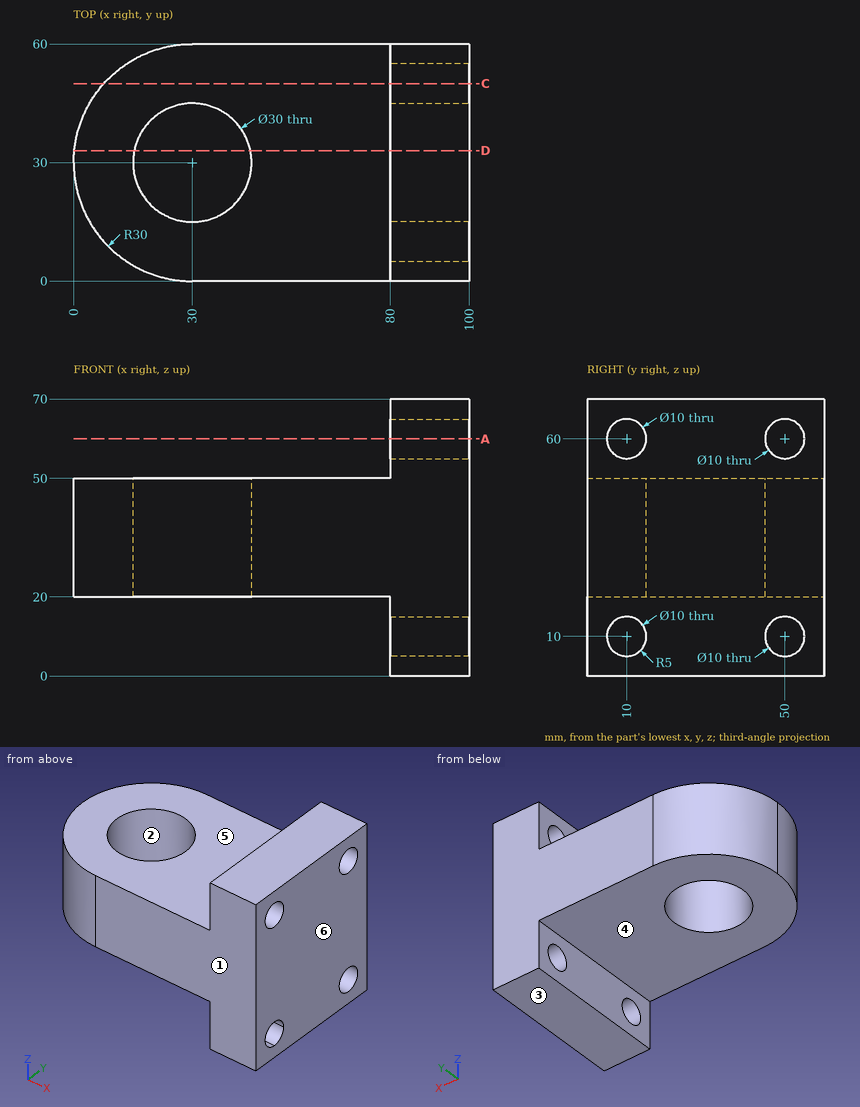
Check sheet for the drawn part. Datum: minimum x, y, z corner. Units: mm. A direction names the side the tool comes from. Coordinates: 2 decimals unless noted, no trailing zeros. Order: outer loops, then holes, each group sorted by start corner. A loop starts at its lowest first (then second) coordinate and runs counter-clockwise, first axis right, second up. Notation, with made-up numbers: (-11, 84.5) -> (8, 84.5) arc R29 cw to (8, 113.5) -> close; hole circle Ø11 at (21, 2). An arc over 180 degrees is marked (long way). Use a Markdown table: item, result. Add a question column.
1. Cross-section at D-D (y = 33). Enter the section's corners in (x, z), and give its area (3 significant figures).
2. Cross-section at A-A (z = 60). Enter the section's corners in (x, y).
3. Mould release check, pull along Y, two halves, no side actions. Record for the marked faces 1, 2 and 3: pulls with the +Y half, pulls with the -Y half, needs draft (parallel to the pull), parting line crosses it, or undercut.
4. Set-up check for the marked faces 4, 5 and 6: record each of +Z, -Z, +X, -X, +Y, -Y from which the full face is reachable in a straight line by a thin tool's end or side.
5. Go/stop test with flat-tipped pins: pin 1 Ø6 at (y, z) = (22, 7.5) entering from -X; pin 2 Ø6 at (x, y) = (54.5, 37) entering from +Z; pin 3 Ø16 at (y, z) = (10, 10) entering from +X; pin 4 Ø10 at (y, z) = (50, 52) entering from -X. Record where each tip stops, or that it passes through.
6. Cross-section at C-C (y = 50). Enter the section's corners in (x, z), and give its area (3 significant figures).
7. Material ranges on L1, parallel to Z at x = 92.5, y = 50; L2, parallel to Y at x = 30, z = 35; L3, parallel to X at y = 54.5, z = 7.5, recorded low to high.
Filled sheet:
| question | item | result |
|---|---|---|
| 1 | outline | (0.15, 20) -> (15.3, 20) -> (15.3, 50) -> (0.15, 50) -> close; (44.7, 20) -> (80, 20) -> (80, 0) -> (100, 0) -> (100, 70) -> (80, 70) -> (80, 50) -> (44.7, 50) -> close |
| 1 | area | 2,910 mm2 |
| 2 | outline | (80, 0) -> (100, 0) -> (100, 5) -> (80, 5) -> close; (80, 15) -> (100, 15) -> (100, 45) -> (80, 45) -> close; (80, 55) -> (100, 55) -> (100, 60) -> (80, 60) -> close |
| 3 | face 1 | pulls with the -Y half |
| 3 | face 2 | undercut |
| 3 | face 3 | needs draft |
| 4 | face 4 | -Z, -X, +Y, -Y |
| 4 | face 5 | +Z, -X, +Y, -Y |
| 4 | face 6 | +Z, -Z, +X, +Y, -Y |
| 5 | pin 1 | x = 80 |
| 5 | pin 2 | z = 50 |
| 5 | pin 3 | x = 100 |
| 5 | pin 4 | x = 4.26 |
| 6 | outline | (7.64, 20) -> (80, 20) -> (80, 15) -> (100, 15) -> (100, 55) -> (80, 55) -> (80, 50) -> (7.64, 50) -> close; (80, 0) -> (100, 0) -> (100, 5) -> (80, 5) -> close; (80, 65) -> (100, 65) -> (100, 70) -> (80, 70) -> close |
| 6 | area | 3,170 mm2 |
| 7 | L1 | 0 to 5, 15 to 55, 65 to 70 |
| 7 | L2 | 0 to 15, 45 to 60 |
| 7 | L3 | 80 to 100 |
